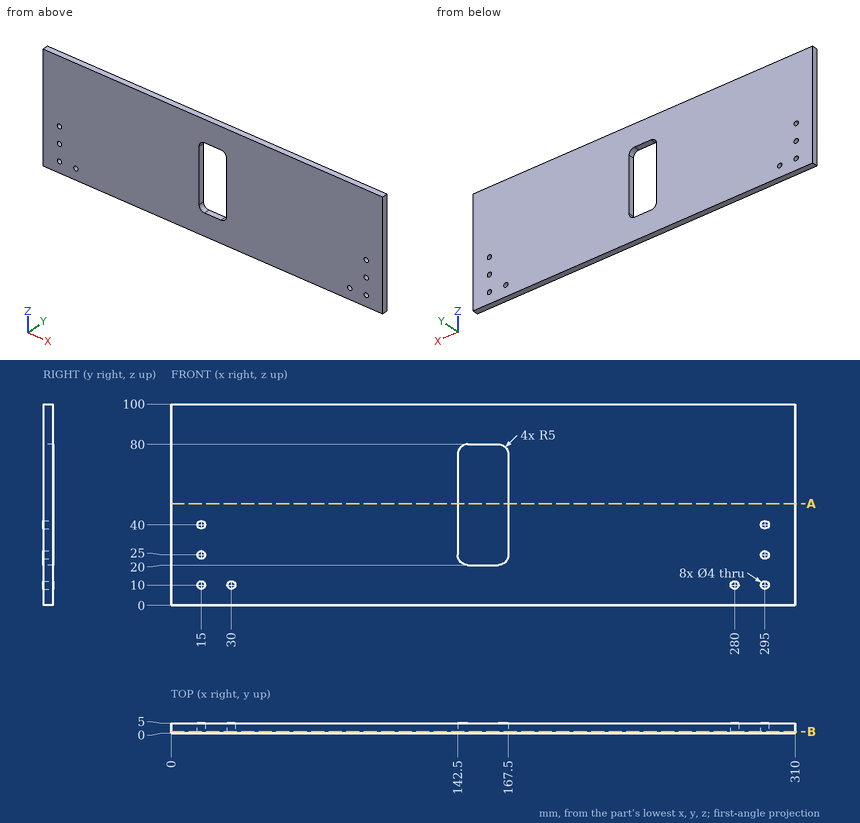
Job drawing, mm, ordinate dimensions from the low corner. One solid piece. Coordinates: 2 decimals unless noted, no trailing zeros. Write each loop counter-clockwise with the first axis right and the second up, starting at its lowest first coordinate (ties: lowest second). Pieces come first, ordered by that corner, then holes. Notation, with made-up numbers: M 34,65 L 82,65 A24 cw 82,96 Z; hole C 44,71 d3. An arc over 180 degrees is marked long. Answer as a JSON object with one key per item and string values. Group by question number.
1) Saw through at B-B (y = 0.85). Give the number of separate pieces and of enclosed holes in the cut face, plus the area to 3 significant figures.
2) Wall check: line 1 (X direction, y = 3.85, z = 10); line 2 (Z direction, x = 295, y = 1.9); line 3 (Z direction, x = 149.5, y = 4). Give the ranges that are in metal, low to high. Write a range as from..to.
3) Saw through at A-A (z = 50.5). Write the cut outline in (x, y).
4) Pin check, flat tips, straight feed: pin 1 Ø2.5 at (x, z) = (15, 40) entering from +Y; pin 2 Ø4.5 at (x, z) = (15, 10) entering from -Y. Stop position of each tip, or through.
Values follow:
{
 "1": {"separate pieces": "1", "enclosed holes": "9", "area": "29,400 mm2"},
 "2": {"line 1": "x = 0..13, 17..28, 32..278, 282..293, 297..310", "line 2": "z = 0..8, 12..23, 27..38, 42..100", "line 3": "z = 0..20, 80..100"},
 "3": {"outline": "M 0,0 L 142.5,0 L 142.5,5 L 0,5 Z; M 167.5,0 L 310,0 L 310,5 L 167.5,5 Z"},
 "4": {"pin 1": "passes through", "pin 2": "stops at y = 0"}
}
